The listing builds one solid part. Answer for the finished solid, in the listing's coordinates (mm). A direction names the side the tool comes from. Coordinates: 2 decimals unless noted, no trailing zeros. Write each loop counter-clockwise with the first axis right and the second up, starting at its lowest first coordinate (ties: lowest second). Pieces come first, ordered by that corner, then holes.
(1) Straight lines are drawn through the part: line 1 (Z direction, x = -28, y = 3); line 2 (Y direction, x = 10, z = 0.6); line 3 (X direction, y = 6, z = 7.5). For each, find the intervals that lie inside material, in ascending order.
(2) For a pull along Z with two mould halves and no side action, classify faces 1 (the flat face through (-32, 0, 6)), 2 (the flat face through (22, -23, 2)), 3 (the flat face through (0.5, 32, 10.6)) as +Z half, -Z half, draft (parallel to the pull), parting line (faces both ways), or undercut.
(3) The part is cut by section B-B on y = -18. Determine the outline of the cut face in (x, z), plus the area to 3 significant figures.
(4) The part is cut by section C-C on x = -31. Determine the outline of the cut face in (y, z), plus the area to 3 significant figures.
(5) The part is cut by section D-D on y = 22. Determine the outline of the cut face in (x, z) (3 decimals), plus the area to 3 significant figures.
(6) Given P1, Ø3.5, axis at x = 32, z = 10.5, coming from the -Y side; P2, Ø1.5, axis at y = -33, z = 10.5, coming from the +X side; P3, Ø0.9, axis at x = -14, z = 9.5, coming from the -Y side (3 decimals), each flat-ended and moving along its own axis, determine where each tip first touches the part or whether it passes through.
(7) Which of the six approach directions +Z, -Z, +X, -X, +Y, -Y give full straight-line access (tool end or side, diameter ignored) to faces 4 (the flat face through (-15, -20.235, 10)), 5 (the conical face through (12.83, -9.37, 1.7)), 6 (the flat face through (-6, 7, 8.6))?
(8) The part is cut by section A-A on x = -15.5. Determine the outline of the cut face in (y, z), plus the area to 3 significant figures.
from build123d import *
from OCP.BRepFilletAPI import BRepFilletAPI_MakeChamfer

# Parameters (mm, degrees)
ESQUISSE1_W             = 70
ESQUISSE1_H             = 70
BOSS_EXTRU_1_DEPTH      = 4
BOSS_EXTRU_2_DEPTH      = 4.6
BOSS_EXTRU_3_DEPTH      = 3
CHANFREIN1_SIZE         = 2
CHANFREIN1_SIZE2        = 6
CHANFREIN2_SIZE         = 25
ENL_V_MAT_EXTRU_1_REACH = 78.476
ESQUISSE6_W             = 67
ESQUISSE6_H             = 4.6


with BuildPart() as part:
    # Esquisse1 → Boss.-Extru.1 (new body)
    with BuildSketch(Plane.XY):
        Rectangle(ESQUISSE1_W, ESQUISSE1_H)
    extrude(amount=BOSS_EXTRU_1_DEPTH)

    # Esquisse2 → Boss.-Extru.2 (add)
    with BuildSketch(Plane.XY.offset(4)):
        Polygon((-35, 35), (-35, -35), (-32, -35), (-32, 32), (35, 32), (35, 35), align=None)
    extrude(amount=BOSS_EXTRU_2_DEPTH)

    # Esquisse3 → Boss.-Extru.3 (add)
    with BuildSketch(Plane.XY.offset(8.6)):
        with BuildLine():
            Line((35, 35), (-35, 35))
            Line((-35, 35), (-35, -35))
            Line((-35, -35), (-27, -35))
            Line((-27, -35), (-27, -30))
            ThreePointArc((-27, -30), (-20.095113441, -27.13990234), (-17.235015781, -20.235015781))
            Line((-17.235015781, -20.235015781), (-12.235015781, -20.235015781))
            ThreePointArc((-12.235015781, -20.235015781), (-2.207811813, 3.972796032), (22, 14))
            Line((22, 14), (22, 19))
            ThreePointArc((22, 19), (27.656854249, 21.343145751), (30, 27))
            Line((30, 27), (35, 27))
            Line((35, 27), (35, 35))
        make_face()
    extrude(amount=BOSS_EXTRU_3_DEPTH)

    # Chanfrein1: one chamfer whose edges measure the first distance from different faces: ONE call of the kernel's chamfer builder (chamfer() names one face for all edges)
    chanfrein1_edges_1 = [part.edges().sort_by_distance(p)[0] for p in [
        (0, 35, 11.6),
    ]]
    chanfrein1_side_1 = [part.faces().sort_by_distance(p)[0] for p in [
        (0, 35, 5.8),
    ]]
    chanfrein1_edges_2 = [part.edges().sort_by_distance(p)[0] for p in [
        (-35, 0, 11.6),
    ]]
    chanfrein1_side_2 = [part.faces().sort_by_distance(p)[0] for p in [
        (-35, 0, 5.8),
    ]]
    chanfrein1 = BRepFilletAPI_MakeChamfer(part.part.solid().wrapped)
    for e in chanfrein1_edges_1:
        chanfrein1.Add(CHANFREIN1_SIZE, CHANFREIN1_SIZE2, e.wrapped, chanfrein1_side_1[0].wrapped)  # the first distance lies on this face
    for e in chanfrein1_edges_2:
        chanfrein1.Add(CHANFREIN1_SIZE, CHANFREIN1_SIZE2, e.wrapped, chanfrein1_side_2[0].wrapped)  # the first distance lies on this face
    add(Compound.cast(chanfrein1.Shape()), mode=Mode.REPLACE)

    # Chanfrein2
    chanfrein2_edges = [part.edges().sort_by_distance(p)[0] for p in [
        (35, -35, 2),
    ]]
    chamfer(chanfrein2_edges, length=CHANFREIN2_SIZE)

    # Esquisse4 → Fraisage pour vis à tête fraisée M51 (revolve, cut)
    with BuildSketch(Plane(origin=(10, -10, 4), x_dir=(0, -1, 0), z_dir=(1, 0, 0))):
        Polygon((0, 0), (0, 4), (2.75, 4), (2.75, 2.45), (5.2, 0), align=None)
    revolve(axis=Axis((10, -10, 10.35), (0, 0, -1)), mode=Mode.SUBTRACT)

    # Esquisse6 → Enlèv. mat.-Extru.1 (cut, up to next)
    with BuildSketch(Plane.XZ.offset(-32), mode=Mode.PRIVATE) as enl_v_mat_extru_1_sk1:
        with Locations((1.5, 6.3)):
            Rectangle(ESQUISSE6_W, ESQUISSE6_H)
    enl_v_mat_extru_1_tool1 = extrude(enl_v_mat_extru_1_sk1.sketch, amount=-ENL_V_MAT_EXTRU_1_REACH, mode=Mode.PRIVATE) & part.part
    add(enl_v_mat_extru_1_tool1.solids().sort_by_distance((1.5, 32, 6.3))[0], mode=Mode.SUBTRACT)


solid = part.part
Model answer:
1. line 1: z = 0 to 4, 8.6 to 11.6
1. line 2: y = -35 to -12.75, -7.25 to 35
1. line 3: x = -35 to -32
2. face 1: undercut
2. face 2: draft
2. face 3: +Z half
3. outline: (-35, 0) - (27, 0) - (27, 4) - (-32, 4) - (-32, 8.6) - (-12.16, 8.6) - (-12.16, 11.6) - (-29, 11.6) - (-35, 9.6) - close
3. area: 324 mm2
4. outline: (-35, 0) - (35, 0) - (35, 4) - (-35, 4) - close; (-35, 8.6) - (35, 8.6) - (35, 9.6) - (31, 10.93) - (-35, 10.93) - close
4. area: 441 mm2
5. outline: (-35, 0) - (35, 0) - (35, 4) - (-32, 4) - (-32, 8.6) - (28.245, 8.6) - (28.245, 11.6) - (-29, 11.6) - (-35, 9.6) - close
5. area: 478 mm2
6. P1: stops at y = 27
6. P2: stops at x = -27
6. P3: stops at y = -20.235
7. face 4: +Z, +X, -Y
7. face 5: +Z
7. face 6: +X, +Y, -Y
8. outline: (-35, 0) - (35, 0) - (35, 4) - (-35, 4) - close; (-20.24, 8.6) - (35, 8.6) - (35, 9.6) - (29, 11.6) - (-20.24, 11.6) - close
8. area: 440 mm2
